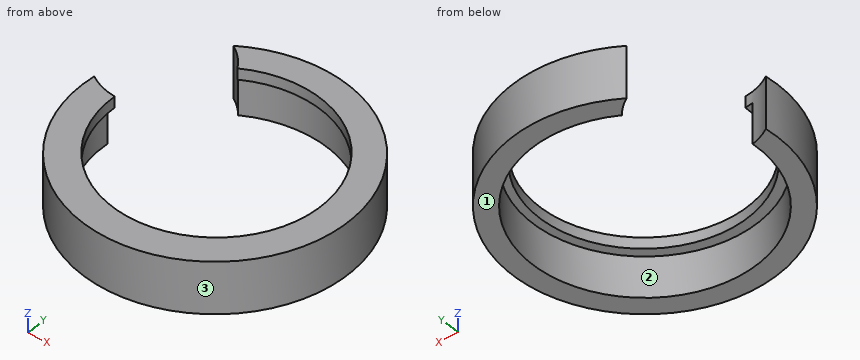
from build123d import *

# Parameters (mm, degrees)
SKETCH_1_R           = 56
SKETCH_1_R_2         = 47.5
EXTRUDE_1_DEPTH      = 20
EXTRUDE_3_DEPTH      = 2
EXTRUDE_3_DEPTH_BACK = 2.7
SKETCH_3_R           = 56
SKETCH_3_R_2         = 44
SKETCH_4_R           = 24
CUT_EXTRUDE_1_DEPTH  = 83.194890352


with BuildPart() as part:
    # 草图1 → 凸台-拉伸1 (new body)
    with BuildSketch(Plane.XY):
        Circle(SKETCH_1_R)
        Circle(SKETCH_1_R_2, mode=Mode.SUBTRACT)
    extrude(amount=EXTRUDE_1_DEPTH)

    # 草图3 → 凸台-拉伸3 (add, two sides: drawn at the far end of the back side and taken through both)
    with BuildSketch(Plane.XY.offset(20).offset(-EXTRUDE_3_DEPTH_BACK)):
        Circle(SKETCH_3_R)
        with Locations((0, 0.69041818)):
            Circle(SKETCH_3_R_2, mode=Mode.SUBTRACT)
    extrude(amount=EXTRUDE_3_DEPTH + EXTRUDE_3_DEPTH_BACK)

    # 草图4 → 切除-拉伸1 (cut, through all)
    with BuildSketch(Plane(origin=(0, 0, 0), x_dir=(-1, 0, 0), z_dir=(0, 0, -1))):
        with Locations((43.301270189, 25)):
            Circle(SKETCH_4_R)
    extrude(amount=-CUT_EXTRUDE_1_DEPTH, mode=Mode.SUBTRACT)


solid = part.part
For this review, take the finished solid that the model builds, in its own axes (mm). Face numbers are marked on the shaded views. Round coordinates to 2 decimals unless told otherwise and drop trailing zeros. Order: outer loops, then holes, each group sorted by start corner. A loop starts at its lowest first (then second) coordinate and runs counter-clockwise, first axis right, second up. Notation, with made-up numbers: (61.25, 33) -> (91.25, 33) arc R9 ccw to (91.25, 48) -> close; hole circle Ø5 at (16.5, 10). An arc over 180 degrees is marked (long way). Write item = value, one per line. Start each with the question number.
1) The part is to be moulded in two halves that separate along X. For the marked faces 1, 2 and 3, say which applies: +X half, -X half, draft (parallel to the pull), parting line (faces both ways), or undercut.
2) To check wall thickness, follow line 1 (Y direction, x = 0, z = 6.5); line 2 (Y direction, x = 26.5, z = 2.5). State the ranges of each line that lie inside material, in increasing order. Write a range as from..to.
3) Take a section at B-B on y = -24. State the section outline as (x, z) points, plus the area to 3 significant figures.
4) Take a section at C-C on y = 34.5. State the section outline as (x, z) points.
5) Insertion check: pin 1 (8 mm diameter, centred on x = 43, z = 18.5, fed in from -Y); pin 2 (6 mm diameter, centred on y = -29, z = 2.5, fed in from -X); pin 3 (5 mm diameter, centred on x = 21, z = 19, fed in from -Y). Each pin has a flat end and moves straight along its axis. Give the tip position at first contact, or say it passes through.
6) Take a section at A-A on x = 0. State the section outline as (y, z) points.
7) Take a section at D-D on x = 45.5. State the section outline as (y, z) points, plus the area to 3 significant figures.
Verdict:
q1.face_1 = draft
q1.face_2 = undercut
q1.face_3 = parting line
q2.line_1 = -56..-47.5, 47.5..56
q2.line_2 = -49.33..-39.42, 39.42..49.33
q3.outline = (-50.6, 0) -> (-40.99, 0) -> (-40.99, 17.3) -> (-36.42, 17.3) -> (-36.42, 22) -> (-50.6, 22) -> close; (36.42, 17.3) -> (40.99, 17.3) -> (40.99, 0) -> (50.6, 0) -> (50.6, 22) -> (36.42, 22) -> close
q3.area = 466 mm2
q4.outline = (28.16, 17.3) -> (32.65, 17.3) -> (32.65, 0) -> (44.11, 0) -> (44.11, 22) -> (28.16, 22) -> close
q5.pin_1 = -40.19
q5.pin_2 = -49.6
q5.pin_3 = -52.86
q6.outline = (-56, 0) -> (-47.5, 0) -> (-47.5, 17.3) -> (-43.31, 17.3) -> (-43.31, 22) -> (-56, 22) -> close; (44.69, 17.3) -> (47.5, 17.3) -> (47.5, 0) -> (56, 0) -> (56, 22) -> (44.69, 22) -> close
q7.outline = (-32.65, 0) -> (-13.64, 0) -> (-13.64, 17.3) -> (13.64, 17.3) -> (13.64, 0) -> (32.65, 0) -> (32.65, 22) -> (-32.65, 22) -> close
q7.area = 965 mm2
